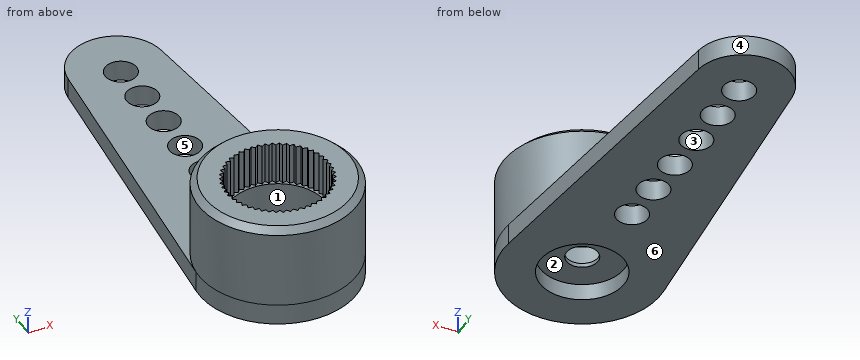
```python
from build123d import *
from build123d.topology import SkipClean

# Parameters (mm, degrees)
BOSS_EXTRUDE1_DEPTH = 1
SKETCH2_R           = 3.75
SKETCH2_R_2         = 2.275
BOSS_EXTRUDE2_DEPTH = 4
SKETCH3_R           = 2
CUT_EXTRUDE1_DEPTH  = 0.8
SKETCH4_R           = 0.75
CUT_EXTRUDE2_DEPTH  = 0.2
SKETCH5_R           = 0.75
CUT_EXTRUDE3_DEPTH  = 1
CHAMFER1_SIZE       = 0.3
CUT_EXTRUDE4_START  = -2
CUT_EXTRUDE4_DEPTH  = 2
CIRPATTERN1_COUNT   = 50


with BuildPart() as part:
    # Sketch1 → Boss-Extrude1 (new body)
    with BuildSketch(Plane.XY):
        with BuildLine():
            Line((-3.731202889, 0.375), (-2.238721733, 15.225))
            ThreePointArc((-2.238721733, 15.225), (0, 17.25), (2.238721733, 15.225))
            Line((2.238721733, 15.225), (3.731202889, 0.375))
            ThreePointArc((3.731202889, 0.375), (0, -3.75), (-3.731202889, 0.375))
        make_face()
    extrude(amount=BOSS_EXTRUDE1_DEPTH)

    # Sketch2 → Boss-Extrude2 (add)
    with SkipClean():  # the faces are left unmerged after this step: merging them gives an invalid solid
        with BuildSketch(Plane.XY.offset(1)):
            with Locations(Location((0, 0, 0), (0, 0, 174.260829523))):
                Circle(SKETCH2_R)
            Circle(SKETCH2_R_2, mode=Mode.SUBTRACT)
        extrude(amount=BOSS_EXTRUDE2_DEPTH)

    # Sketch3 → Cut-Extrude1 (cut)
    with SkipClean():  # the faces are left unmerged after this step: merging them gives an invalid solid
        with BuildSketch(Plane(origin=(0, 0, 0), x_dir=(-1, 0, 0), z_dir=(0, 0, -1))):
            Circle(SKETCH3_R)
        extrude(amount=-CUT_EXTRUDE1_DEPTH, mode=Mode.SUBTRACT)

    # Sketch4 → Cut-Extrude2 (cut)
    with SkipClean():  # the faces are left unmerged after this step: merging them gives an invalid solid
        with BuildSketch(Plane(origin=(0, 0, 0.8), x_dir=(-1, 0, 0), z_dir=(0, 0, -1))):
            Circle(SKETCH4_R)
        extrude(amount=-CUT_EXTRUDE2_DEPTH, mode=Mode.SUBTRACT)

    # Sketch5 → Cut-Extrude3 (cut)
    with SkipClean():  # the faces are left unmerged after this step: merging them gives an invalid solid
        with BuildSketch(Plane(origin=(0, 0, 0), x_dir=(-1, 0, 0), z_dir=(0, 0, -1))):
            with Locations((0, 4.65)):
                Circle(SKETCH5_R)
            with Locations((0, 6.65)):
                Circle(SKETCH5_R)
            with Locations((0, 8.65)):
                Circle(SKETCH5_R)
            with Locations((0, 10.65)):
                Circle(SKETCH5_R)
            with Locations((0, 12.65)):
                Circle(SKETCH5_R)
            with Locations((0, 14.65)):
                Circle(SKETCH5_R)
        extrude(amount=-CUT_EXTRUDE3_DEPTH, mode=Mode.SUBTRACT)

    # Chamfer1
    chamfer1_edges = [part.edges().sort_by_distance(p)[0] for p in [
        (3.731202889, -0.375, 5),
    ]]
    chamfer(chamfer1_edges, length=CHAMFER1_SIZE)

    # Sketch7 → Cut-Extrude4 (cut)
    with SkipClean():  # the faces are left unmerged after this step: merging them gives an invalid solid
        with BuildSketch(Plane.XY.offset(5).offset(CUT_EXTRUDE4_START)):
            with BuildLine():
                Line((0.147557721, 2.345362812), (0, 2.5))
                Line((0, 2.5), (-0.147557721, 2.345362812))
                Line((-0.147557721, 2.345362812), (-0.142848432, 2.270510807))
                ThreePointArc((-0.142848432, 2.270510807), (0, 2.275), (0.142848432, 2.270510807))
                Line((0.142848432, 2.270510807), (0.147557721, 2.345362812))
            make_face()
        cut_extrude4 = extrude(amount=CUT_EXTRUDE4_DEPTH, mode=Mode.SUBTRACT)

    # CirPattern1: Cut-Extrude4 ×50 about axis
    with SkipClean():  # the faces are left unmerged after this step: merging them gives an invalid solid
        cirpattern1_axis = Axis((0, 0, 0), (0, 0, 1))
        for i in range(1, CIRPATTERN1_COUNT):
            add(cut_extrude4.rotate(cirpattern1_axis, i * 360 / CIRPATTERN1_COUNT), mode=Mode.SUBTRACT)


solid = part.part
```
Here's how the part is built. I have some questions about the finished solid (model axes, mm). Face numbers are marked on the shaded views. A direction names the side the tool comes from. Coordinates: 2 decimals unless noted, no trailing zeros. Loops run counter-clockwise (first coordinate to the right, second up) from the corner with the lowest first, then second, coordinate; pieces in that order, holes last. Notation, with made-up numbers: (-12.5, 28.25) -> (44.5, 28.25) arc R18 cw to (44.5, 55.25) -> close; hole circle Ø4 at (-12.75, 6). An arc over 180 degrees is marked (long way). Return JSON: item names as keys, results as strings.
1) If we section it at A-A, the plane y = 14.65: Write out the boundary of the cut face in (x, z), then the cut area to 3 significant figures.
Results below:
{"outline": "(-2.3, 0) -> (-0.75, 0) -> (-0.75, 1) -> (-2.3, 1) -> close; (0.75, 0) -> (2.3, 0) -> (2.3, 1) -> (0.75, 1) -> close", "area": "3.09 mm²"}
2) Thinking about a two-plate mould opening in Y: for the marked faces 4, 5 and 6, which applies, +Y half, -Y half, draft (parallel to the pull), parting line (faces both ways), or undercut?
Results below:
{"face 4": "+Y half", "face 5": "undercut", "face 6": "draft"}
3) Will these pins go through, and if not, where does the flat tip stop? pin 1 (1.5 mm diameter, centred on x = 0, y = 0.5, fed in from +Z); pin 2 (2 mm diameter, centred on x = 0, y = 4.65, fed in from +Z); pin 3 (2 mm diameter, centred on x = 0.5, y = 0, fed in from -Z).
Results below:
{"pin 1": "z = 1", "pin 2": "z = 4.8", "pin 3": "z = 0.8"}
4) If we section it at B-B, the plane z = 1.25: Write out the boundary of the cut face in (x, y) (3 decimals).
Results below:
{"outline": "circle Ø7.5 at (0, 0); hole circle Ø4.55 at (0, 0)"}
5) If we section it at C-C, the plane y = 8.65: Write out the boundary of the cut face in (x, z).
Results below:
{"outline": "(-2.9, 0) -> (-0.75, 0) -> (-0.75, 1) -> (-2.9, 1) -> close; (0.75, 0) -> (2.9, 0) -> (2.9, 1) -> (0.75, 1) -> close"}
6) For the marked faces 1, 2 and 3, which set-ups out of +Z, -Z, +X, -X, +Y, -Y let a thin tool reach every point of the face, with its end or its side?
Results below:
{"face 1": "+Z", "face 2": "-Z", "face 3": "+Z, -Z"}
7) I need wall thicknesses on line 1 (Z direction, x = -0.5, y = 16); line 2 (Z direction, x = -2.25, y = 0.5); line 3 (X direction, y = 1.75, z = 0.55). Which ranges of each line are inside material? Lowest first, please. Write a range as from..to.
Results below:
{"line 1": "0..1", "line 2": "0..3", "line 3": "-3.59..-0.97, 0.97..3.59"}
